Source: CAD feature listing. Evaluate the final solid. Frame: model axes, mm. A direction names the side the tool comes from. Round coordinates to 2 decimals unless told otherwise and drop trailing zeros. Write each loop counter-clockwise with the first axis right and the second up, starting at its lowest first coordinate (ties: lowest second). Pieces come first, ordered by that corner, then holes. Notation, with made-up numbers: M 84,41.25 L 108,41.25 A12 cw 108,47.25 Z; hole C -26.75,34 d9. An arc over 180 degrees is marked long. Answer in a Markdown table with one row per item.
from build123d import *

# Parameters (mm, degrees)
BOSS_EXTRUDE1_DEPTH = 30
CUT_EXTRUDE1_DEPTH  = 60
CUT_EXTRUDE2_DEPTH  = 60
BOSS_EXTRUDE2_DEPTH = 6
SKETCH6_R           = 7.5
CUT_EXTRUDE3_DEPTH  = 12
SKETCH7_R           = 7.5
CUT_EXTRUDE4_DEPTH  = 12


with BuildPart() as part:
    # Sketch2 → Boss-Extrude1 (new body, symmetric)
    with BuildSketch(Plane.XY):
        Polygon((100, 0), (0, 0), (-40, 69.282032303), (-31.339745962, 74.282032303), (5.773502692, 10), (100, 10), align=None)
    extrude(amount=BOSS_EXTRUDE1_DEPTH, both=True)

    # Sketch3 → Cut-Extrude1 (cut)
    with BuildSketch(Plane(origin=(0, 10, 0), x_dir=(1, 0, 0), z_dir=(0, 1, 0))):
        with BuildLine():
            ThreePointArc((70, 30), (91.213203452, 21.213203419), (100, -4.6e-08))
            Line((100, -4.6e-08), (100, 30))
            Line((100, 30), (70, 30))
        make_face()
        with BuildLine():
            Line((70, -30), (100, -30))
            Line((100, -30), (100, -4.6e-08))
            ThreePointArc((100, -4.6e-08), (91.213203419, -21.213203452), (70, -30))
        make_face()
    extrude(amount=-CUT_EXTRUDE1_DEPTH, mode=Mode.SUBTRACT)

    # Sketch4 → Cut-Extrude2 (cut)
    with BuildSketch(Plane(origin=(8.660254038, 5, 0), x_dir=(0, 0, -1), z_dir=(0.866025404, 0.5, 0))):
        with BuildLine():
            ThreePointArc((-30, 50), (-21.213203436, 71.213203436), (0, 80))
            Line((0, 80), (-30, 80))
            Line((-30, 80), (-30, 50))
        make_face()
        with BuildLine():
            ThreePointArc((0, 80), (21.213203436, 71.213203436), (30, 50))
            Line((30, 50), (30, 80))
            Line((30, 80), (0, 80))
        make_face()
    extrude(amount=-CUT_EXTRUDE2_DEPTH, mode=Mode.SUBTRACT)

    # Sketch5 → Boss-Extrude2 (add, symmetric)
    with BuildSketch(Plane.XY):
        Polygon((5.773502692, 10), (65.773502692, 10), (-14.226497308, 44.641016151), align=None)
    extrude(amount=BOSS_EXTRUDE2_DEPTH, both=True)

    # Sketch6 → Cut-Extrude3 (cut)
    with BuildSketch(Plane(origin=(0, 10, 0), x_dir=(1, 0, 0), z_dir=(0, 1, 0))):
        with Locations((82.951530003, 0)):
            Circle(SKETCH6_R)
    extrude(amount=-CUT_EXTRUDE3_DEPTH, mode=Mode.SUBTRACT)

    # Sketch7 → Cut-Extrude4 (cut)
    with BuildSketch(Plane(origin=(0, 0, 0), x_dir=(0, 0, 1), z_dir=(-0.866025404, -0.5, 0))):
        with Locations((0, 64.952644295)):
            Circle(SKETCH7_R)
    extrude(amount=-CUT_EXTRUDE4_DEPTH, mode=Mode.SUBTRACT)


solid = part.part
Q1. Section C-C (y = 6). Return loops of the section in (x, z), and give its area (3 significant figures).
Solutions:
| item | result |
|---|---|
| outline | M -3.46,-30 L 70,-30 A30 ccw 70,30 L -3.46,30 Z; hole C 82.95,0 d15 |
| area | 5,640 mm2 |
Q2. Material intervals for probe 1 along Z at (x, y) = (4, 32.5); probe 2 along Y at (x, z) = (38.5, 14.5); probe 3 along Y at (x, z) = (-8, -9.5), sorted ascending.
Solutions:
| item | result |
|---|---|
| probe 1 | z = -6 to 6 |
| probe 2 | y = 0 to 10 |
| probe 3 | y = 13.86 to 33.86 |
Q3. Section D-D (z = 26.5). Return loops of the section in (x, y).
Solutions:
| item | result |
|---|---|
| outline | M -32.03,55.48 L 0,0 L 84.06,0 L 84.06,10 L 5.77,10 L -23.37,60.48 Z |
Q4. Pull-direction query (X, two-part tool) for faces 1 (the flat face through (-13.043, 42.591, 7.087)), 2 (the flat face through (-19.72, 34.16, 0.42)), 3 (the cylindrical face through (75.46, 5.07, -0.33)), 4 (the flat face through (23, 8, -30)); classes: pulls with the +X half, pulls with the -X half, needs draft (parallel to the pull), parting line crosses it, or undercut.
Solutions:
| item | result |
|---|---|
| face 1 | pulls with the +X half |
| face 2 | pulls with the -X half |
| face 3 | undercut |
| face 4 | needs draft |
Q5. Contact query for flat-ended pins moving along their axis: pin 1 Ø6 at (x, y) = (-22.5, 47.5) entering from +Z; pin 2 Ø12 at (y, z) = (24.5, -4) entering from -X; pin 3 Ø12 at (x, z) = (82.95, 0) entering from +Y; pin 4 Ø8 at (x, y) = (16.5, 22) entering from -Z. Output: stop coordinate, or through.
Solutions:
| item | result |
|---|---|
| pin 1 | stops at z = 30 |
| pin 2 | stops at x = -17.61 |
| pin 3 | passes through |
| pin 4 | stops at z = -6 |
Q6. Section B-B (z = -13). Return loops of the section in (x, y).
Solutions:
| item | result |
|---|---|
| outline | M -38.52,66.72 L 0,0 L 97.04,0 L 97.04,10 L 5.77,10 L -29.86,71.72 Z |
Q7. Section A-A (y = 24). Return loops of the section in (x, z), and give its area (3 significant figures).
Solutions:
| item | result |
|---|---|
| outline | M -13.86,-30 L -2.31,-30 L -2.31,-6 L 33.44,-6 L 33.44,6 L -2.31,6 L -2.31,30 L -13.86,30 Z |
| area | 1,120 mm2 |
Q8. Access query for faces 5 (the flat face through (52.2, 10, -6.2)), 6 (the flat face through (20, 21, -6)), 7 (the flat face through (20, 21, 6)). Directions: +Z, -Z, +X, -X, +Y, -Y. A direction counts if a zero-diameter tool reaches every point of the face in a straight line with its end or side. Return the directions, or none.
Solutions:
| item | result |
|---|---|
| face 5 | +X, +Y |
| face 6 | -Z, +X, +Y |
| face 7 | +Z, +X, +Y |
